Autodesk Inventor part; units mm, degrees
ref_plane "YZ Plane" through (0, 0, 0) normal (1, 0, 0) x (0, 1, 0)
ref_plane "XZ Plane" through (0, 0, 0) normal (0, 1, 0) x (-1, 0, 0)
ref_plane "XY Plane" through (0, 0, 0) normal (0, 0, 1) x (1, 0, 0)
sketch "Sketch1" plane through (0, 0, 0) normal (0, 0, 1) x (1, 0, 0)
  line L0 (0, 0) -> (0, 130)
  line L1 (-54, 0) -> (-54, 31.5294)
  line L2 (-79.5, 98.4706) -> (-79.5, 130)
  line L3 (-79.5, 130) -> (-75, 130)
  line L4 (-75, 130) -> (-75, 98.4706)
  line L5 (-50, 31.5294) -> (-50, 0)
  line L6 (-73.5135, 76.4935) -> (-59.9865, 53.5065)
  line L7 (-69.0135, 76.4935) -> (-56.4175, 55.0885)
  arc A0 (-75, 98.4706) -> (-69.0135, 76.4935) centre (-31.6667, 98.4706) ccw
  arc A1 (-79.5, 98.4706) -> (-73.5135, 76.4935) centre (-36.1667, 98.4706) ccw
  arc A2 (-54, 31.5294) -> (-59.9865, 53.5065) centre (-97.3333, 31.5294) ccw
  arc A3 (-50, 31.5294) -> (-56.4175, 55.0885) centre (-96.4526, 31.5294) ccw
  line L8 (-54, 0) -> (-50, 0)
  point P0 (-54, 43.3333)
  point P1 (-79.5, 86.6667)
  point P2 (-77.25, 130)
  point P3 (-52, 0)
  dimension "d0" = 4
  dimension "d1" = 108
  dimension "d2" = 4.5
  dimension "d3" = 159
  dimension "d5" = 43.3333
  dimension "d6" = 43.3333
  dimension "d8" = 43.3333
  dimension "d13" = 130
  dimension "d15" = 43.3333
revolve "Revolution1" add sketch "Sketch1" angle 360 about axis through (0, 0, 0) along (0, 1, 0)
equation "\"d0\" = s1"
equation "\"d1\" = dh_"
equation "\"d2\" = s_"
equation "\"d3\" = Dh"
equation "\"d8\" = 0.333333 * L"
equation "\"d13\" = L"
equation "\"d15\" = 0.333333 * L"
equation "\"L\" = 130"
equation "\"s_\" = 4.5"
equation "\"Dh\" = 159"
equation "\"dh_\" = 108"
equation "\"s1\" = 4"
properties part number "Reducer К 159x4.5-108x4 GOST 17378-83" material "Steel, Mild"
Check sheet for the modelled part. Datum: model origin and axes. Units: mm. A direction names the side the tool comes from. Round coordinates to 2 decimals unless told otherwise and drop trailing zeros. Order: outer loops, then holes, each group sorted by start corner. A loop starts at its lowest first (then second) coordinate and runs counter-clockwise, first axis right, second up. Notation, with made-up numbers: (17, 33.5) -> (38, 33.5) arc R5 ccw to (38, 37.5) -> close; hole circle Ø7 at (22.25, -25.5). An arc over 180 degrees is marked (long way). One line per item, written item: value. Start each with the question number.
Q1. Cross-section at A-A (y = 61.5). Record the boundary of the cut face in (x, z).
Q2. Gauge pin test, flat ends, axial feed: pin 1 Ø3 at (y, z) = (106, 10.5) entering from +X; pin 2 Ø6 at (x, y) = (-4.5, 38.5) entering from +Z; pin 3 Ø8 at (x, y) = (-17.5, 13) entering from -Z. Record the tip position at first contact, or that the pin passes through.
Q3. Mould release check, pull along Z, two halves, no side actions. Record for faces 3 (the face through (-47.69, 15.54, -15.02)), 4 (the face through (9.764, 114.015, -74.362)), 5 (the face through (-58.02, 54.94, 18.27)), 6 (the face through (-48, 0, -16)): pulls with the +Z half, pulls with the -Z half, needs draft (parallel to the pull), parting line crosses it, or undercut.
Q4. Set-up check for faces 1 (the face through (47, 130, -59)), 2 (the face through (11.706, 15.985, -52.716)): record each of +Z, -Z, +X, -X, +Y, -Y from which the full face is reachable in a straight line by a thin tool's end or side.
Q5. Thickness scan on line 1 (Z direction, x = 0, y = 117); line 2 (Z direction, x = 0, y = 25); line 3 (X direction, y = 110, z = 62). Record the ranges inside material, lowest first.
Completed:
1. outline: circle Ø129.38 at (0, 0); hole circle Ø120.38 at (0, 0)
2. pin 1: stops at x = 78.99
2. pin 2: stops at z = 55.01
2. pin 3: stops at z = -52.29
3. face 3: undercut
3. face 4: undercut
3. face 5: parting line crosses it
3. face 6: needs draft
4. face 1: +Z, -Z, +X, -X, +Y
4. face 2: -Y
5. line 1: z = -79.5 to -75, 75 to 79.5
5. line 2: z = -54 to -50, 50 to 54
5. line 3: x = -49.76 to -42.2, 42.2 to 49.76
